Model file for the job. Use its own axes, mm. Face numbers are marked on the shaded views. A direction names the side the tool comes from. Coordinates: 2 decimals unless noted, no trailing zeros. Order: outer loops, then holes, each group sorted by start corner. A loop starts at its lowest first (then second) coordinate and runs counter-clockwise, first axis right, second up.
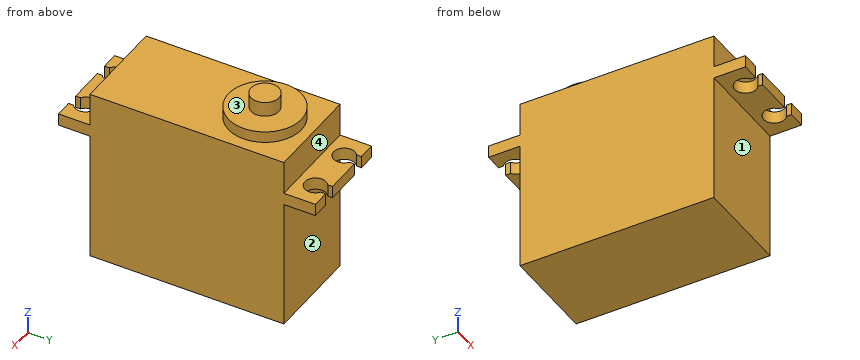
Autodesk Fusion 360 part; units mm, degrees
sketch "Sketch1" plane through (0, 0, 0) normal (0, 0, 1) x (1, 0, 0)
  line L0 (0, 0) -> (19.82, 0)
  line L1 (19.82, 0) -> (19.82, 39.88)
  line L2 (19.82, 39.88) -> (0, 39.88)
  line L3 (0, 39.88) -> (0, 0)
  line L4 (0, 46.36) -> (19.82, 46.36)
  line L5 (19.82, 46.36) -> (19.82, -6.48)
  line L6 (19.82, -6.48) -> (0, -6.48)
  line L7 (0, -6.48) -> (0, 46.36)
  line L8 (9.91, 39.88) -> (9.91, 0) construction
  line L9 (19.82, 19.94) -> (0, 19.94) construction
  circle A0 centre (4.825, 43.57) radius 2.19
  circle A1 centre (14.995, 43.57) radius 2.19
  circle A2 centre (4.825, -3.69) radius 2.19
  circle A3 centre (14.995, -3.69) radius 2.19
  line L10 (3.575, 46.36) -> (3.575, 45.3682)
  line L11 (6.075, 46.36) -> (6.075, 45.3682)
  line L12 (13.745, 46.36) -> (13.745, 45.3682)
  line L13 (16.245, 46.36) -> (16.245, 45.3682)
  line L14 (3.575, -6.48) -> (3.575, -5.4882)
  line L15 (6.075, -6.48) -> (6.075, -5.4882)
  line L16 (13.745, -6.48) -> (13.745, -5.4882)
  line L17 (16.245, -6.48) -> (16.245, -5.4882)
  point P0 (4.825, 43.57)
  point P1 (14.995, 43.57)
  point P2 (4.825, -3.69)
  point P3 (14.995, -3.69)
  dimension "d1" = 19.82
  dimension "d2" = 39.88
  dimension "d3" = 52.84
  dimension "d4" = 47.26
  dimension "d5" = 10.17
  dimension "d15" = 4.38
  dimension "d16" = 2.5
  dimension "d17" = 2.5
extrude "Extrude1" add sketch "Sketch1" along normal blind 9.35 and the other way blind 26.67 contours L0 L1 L2 L3 L5 L7
extrude "Extrude2" add sketch "Sketch1" along normal blind 2.5 contours L0 L5 L6 L7 A2 A3 L14 L15 L16 L17 | L2 L4 L5 L7 A0 A1 L10 L11 L12 L13
sketch "Sketch3" plane through (0, 0, 9.35) normal (0, 0, 1) x (-1, 0, 0)
  line L0 (-19.82, -39.88) -> (0, -39.88)
  line L1 (0, -39.88) -> (0, 0)
  line L2 (0, 0) -> (-19.82, 0)
  line L3 (-19.82, 0) -> (-19.82, -39.88)
  circle A0 centre (-9.91, -30.22) radius 7.5
  circle A1 centre (-9.91, -30.22) radius 2.88
  line L4 (-9.91, -39.88) -> (-9.91, -30.22) construction
  dimension "d19" = 9.66
  dimension "d20" = 15
  dimension "d21" = 5.76
extrude "Extrude3" add sketch "Sketch3" along normal blind 2.33 contours A0
extrude "Extrude4" add sketch "Sketch3" along normal blind 5.38 contours A1
equation "d4 = 13.47 mm + 33.79 mm"
equation "d21 = ( 2.88 * 2 ) * 1 mm"
equation "d22 = 11.68 mm - 9.35 mm"
equation "d24 = 11.68 mm - 9.35 mm + 3.05 mm"
Q1. Cut at D-D, the plane z = -17. List the corners of the cut face in (x, y), plus the area to 3 significant figures.
Established:
outline: (0, 0) - (19.82, 0) - (19.82, 39.88) - (0, 39.88) - close
area: 790 mm2
Q2. Cut at C-C, the plane y = 30.22. List the corners of the cut face in (x, z).
Established:
outline: (0, -26.67) - (19.82, -26.67) - (19.82, 9.35) - (17.41, 9.35) - (17.41, 11.68) - (12.79, 11.68) - (12.79, 14.73) - (7.03, 14.73) - (7.03, 11.68) - (2.41, 11.68) - (2.41, 9.35) - (0, 9.35) - close
Q3. Which spindle directions (+Z, -Z, +X, -X, +Y, -Y) get a long thin tool onto all of the face, cutting with end or side? Do the marked faces 1, 2, 3 and 4. Say none if no direction does.
Established:
face 1: -Z, +X, -X, -Y
face 2: -Z, +X, -X, +Y
face 3: +Z
face 4: +Z, +X, -X, +Y
Q4. Drop flat-ended pins along their axis: P1, Ø3, axis at x = 12.5, y = -5, coming from the +Z side; P2, Ø4, axis at x = 12, z = 10.5, coming from the -Y side; P3, Ø1.9, axis at x = 9, y = 42, coming from the -Z side. Give the stop position or say it passes through.
Established:
P1: stops at z = 2.5
P2: stops at y = 0
P3: stops at z = 0
Q5. Cut at A-A, the plane y = 43.57. List the corners of the cut face in (x, z) (3 decimals).
Established:
outline: (0, 0) - (2.635, 0) - (2.635, 2.5) - (0, 2.5) - close; (7.015, 0) - (12.805, 0) - (12.805, 2.5) - (7.015, 2.5) - close; (17.185, 0) - (19.82, 0) - (19.82, 2.5) - (17.185, 2.5) - close
Q6. Cut at B-B, the plane x = 9.91. List the corners of the cut face in (y, z).
Established:
outline: (-6.48, 0) - (0, 0) - (0, -26.67) - (39.88, -26.67) - (39.88, 0) - (46.36, 0) - (46.36, 2.5) - (39.88, 2.5) - (39.88, 9.35) - (37.72, 9.35) - (37.72, 11.68) - (33.1, 11.68) - (33.1, 14.73) - (27.34, 14.73) - (27.34, 11.68) - (22.72, 11.68) - (22.72, 9.35) - (0, 9.35) - (0, 2.5) - (-6.48, 2.5) - close
Q7. Probe line 1 (X direction, y = 43.57, z = 1.7) (3 decimals); line 2 (Y direction, x = 16.75, z = 0.5); line 3 (Z direction, x = 13, y = 38). List the from-to ranges inside material, lowest first.
Established:
line 1: x = 0 to 2.635, 7.015 to 12.805, 17.185 to 19.82
line 2: y = -6.48 to -5, -2.38 to 42.26, 44.88 to 46.36
line 3: z = -26.67 to 9.35
